Read the model definition and answer for the solid it produces. Units are mm, in the model's axes. A direction names the side the tool comes from. Coordinates: 2 decimals unless noted, no trailing zeros. Write each loop counter-clockwise with the first axis right and the second up, starting at its lowest first coordinate (ties: lowest second). Pieces come first, ordered by that corner, then holes. Notation, with made-up numbers: (11, 21.5) - (39, 21.5) arc R29 cw to (39, 53.5) - close; hole circle Ø1 at (87, 31.25). An arc over 180 degrees is marked (long way). Return JSON: item names as keys, results as strings.
```python
from build123d import *

# Parameters (mm, degrees)
F0_W     = 76.2
F0_H     = 38.1
F1_DEPTH = 25.4
F2_W     = 5.08
F2_H     = 5.08
F3_DEPTH = 5.08
F4_W     = 62.375739
F4_H     = 17.19705
F5_DEPTH = 25.4


with BuildPart() as f1:
    # F0 (on Front) → F1 (new body)
    with BuildSketch(Plane.XZ):
        with Locations((38.1, -19.05)):
            Rectangle(F0_W, F0_H)
    extrude(amount=F1_DEPTH)

    # F2 (on face) → F3 (join)
    with BuildSketch(Plane(origin=(0, 0, -38.1), x_dir=(1, 0, 0), z_dir=(0, 0, -1))):
        with Locations((2.54, 22.86)):
            Rectangle(F2_W, F2_H)
        with Locations((2.54, 2.54)):
            Rectangle(F2_W, F2_H)
        with Locations((73.66, 22.86)):
            Rectangle(F2_W, F2_H)
        with Locations((73.66, 2.54)):
            Rectangle(F2_W, F2_H)
    extrude(amount=F3_DEPTH)

    # F4 (on face) → F5 (cut)
    with BuildSketch(Plane(origin=(0, 0, -38.1), x_dir=(1, 0, 0), z_dir=(0, 0, -1))):
        with Locations((38.183279, 12.533443)):
            Rectangle(F4_W, F4_H)
    extrude(amount=-F5_DEPTH, mode=Mode.SUBTRACT)


solid = f1.part
```
(1) A cutting plane is placed at B-B (y = -2.5). Determine the outline of the cut face in (x, z), and give its area (3 significant figures).
Answer:
{"outline": "(0, -43.18) - (5.08, -43.18) - (5.08, -38.1) - (71.12, -38.1) - (71.12, -43.18) - (76.2, -43.18) - (76.2, 0) - (0, 0) - close", "area": "2,950 mm²"}
(2) A cutting plane is placed at C-C (x = 55). Determine the outline of the cut face in (y, z).
Answer:
{"outline": "(-25.4, -38.1) - (-21.13, -38.1) - (-21.13, -12.7) - (-3.93, -12.7) - (-3.93, -38.1) - (0, -38.1) - (0, 0) - (-25.4, 0) - close"}
(3) A cutting plane is placed at A-A (z = -35.5). Determine the outline of the cut face in (x, y).
Answer:
{"outline": "(0, -25.4) - (76.2, -25.4) - (76.2, 0) - (0, 0) - close; hole (7, -21.13) - (69.37, -21.13) - (69.37, -3.93) - (7, -3.93) - close"}
(4) Straight lines are drawn through the part: line 1 (X direction, y = -15.75, z = -36); line 2 (Y direction, x = 29.5, z = -28.5); line 3 (Z direction, x = 5, y = -8.75). For each, find the intervals that lie inside material, in ascending order. Write a range as from..to.
Answer:
{"line 1": "0..7, 69.37..76.2", "line 2": "-25.4..-21.13, -3.93..0", "line 3": "-38.1..0"}
(5) Which of the six approach directions +Z, -Z, +X, -X, +Y, -Y give full straight-line access (tool end or side, diameter ignored) to faces 5 (the face through (38, -13, 0)), 6 (the face through (38, -3.935, -26)), 7 (the face through (74, -20.32, -41)), 8 (the face through (5.08, -3, -41)), 9 (the face through (74, -3, -43.18))?
Answer:
{"face 5": "+Z, +X, -X, +Y, -Y", "face 6": "-Z", "face 7": "-Z, +X, -X", "face 8": "-Z, +Y, -Y", "face 9": "-Z, +X, -X, +Y, -Y"}
(6) Determine the mould class of faces 1 (the face through (5.08, -23, -41)), 2 (the face through (38, -21.132, -26)), 3 (the face through (74, -23, -43.18)), 4 (the face through (0, -13, -21)) for opening direction X: +X half, -X half, draft (parallel to the pull), parting line (faces both ways), or undercut.
Answer:
{"face 1": "undercut", "face 2": "undercut", "face 3": "draft", "face 4": "-X half"}
(7) A flat-ended cylindrical pin translates along its axis: P1, Ø6, axis at x = 58, y = -7.5, coming from the -Z side. Find the tip coordinate at first contact, or state that the pin passes through.
Answer:
{"P1": "z = -12.7"}
